from build123d import *

# Parameters (mm, degrees)
SKETCH1_W            = 70
SKETCH1_H            = 50
BOSS_EXTRUDE1_DEPTH  = 5
BOSS_EXTRUDE2_DEPTH  = 5
MIRROR2_COPY_1_DEPTH = 5


with BuildPart() as part:
    # Sketch1 → Boss-Extrude1 (new body)
    with BuildSketch(Plane.XY):
        Rectangle(SKETCH1_W, SKETCH1_H)
    extrude(amount=BOSS_EXTRUDE1_DEPTH)

    # Sketch2 → Boss-Extrude2 (add)
    with BuildSketch(Plane.ZY.offset(35)):
        Polygon((3.843440475, -25), (-7.895535709, -41.369324188), (-14.361094855, -42.788640383), (-29.004505052, -42.788640383), (-34.365162286, -38.4026481), (-35, -35), (-29.677149334, -39.79641498), (-19.61481892, -39.79641498), (-9.962095697, -37.111555615), (0, -24.21921522), align=None)
    boss_extrude2 = extrude(amount=-BOSS_EXTRUDE2_DEPTH)

    # Mirror1: Boss-Extrude2 across plane
    add(boss_extrude2.mirror(Plane.ZX))

    # Mirror2: Boss-Extrude2 across plane
    add(boss_extrude2.mirror(Plane(origin=(0, 0, 0), x_dir=(0, 0, 1), z_dir=(1, 0, 0))))

    # Mirror2 copy 1 sketch → Mirror2 copy 1 (add)
    with BuildSketch(Plane(origin=(35, 0, 0), x_dir=(0, 0, 1), z_dir=(1, 0, 0))):
        Polygon((3.843440475, -25), (-7.895535709, -41.369324188), (-14.361094855, -42.788640383), (-29.004505052, -42.788640383), (-34.365162286, -38.4026481), (-35, -35), (-29.677149334, -39.79641498), (-19.61481892, -39.79641498), (-9.962095697, -37.111555615), (0, -24.21921522), align=None)
    extrude(amount=-MIRROR2_COPY_1_DEPTH)


solid = part.part
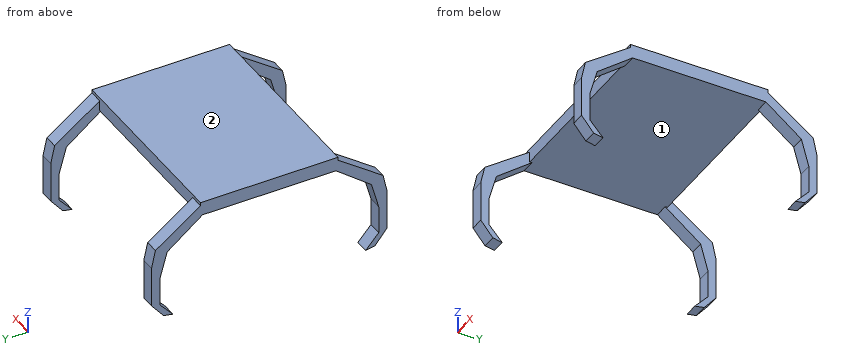
Model file for the job. Use its own axes, mm. Face numbers are marked on the shaded views. Coordinates: 2 decimals unless noted, no trailing zeros. Order: outer loops, then holes, each group sorted by start corner. A loop starts at its lowest first (then second) coordinate and runs counter-clockwise, first axis right, second up. Notation, with made-up numbers: M 2,-35 L 53,-35 A22 cw 53,-15 Z; hole C -23,-32 d5. An arc over 180 degrees is marked long. Return JSON: item names as keys, results as strings.
1. Flat gauge pins, fed straight in: pin 1 (1.5 mm diameter, centred on x = 5, z = 2, fed in from +Y); pin 2 (5.5 mm diameter, centred on x = 8.5, z = 3, fed in from -Y); pin 3 (8 mm diameter, centred on x = 15, y = -28.5, fed in from -Z). Where does each tip first touch, or does it go through?
Ans:
{"pin 1": "y = 25", "pin 2": "y = -25", "pin 3": "z = 0"}
2. Saw through at D-D (z = -9). Give the cut face in (x, y), and give its area (3 significant figures).
Ans:
{"outline": "M -35,-41.61 L -30,-41.61 L -30,-35.87 L -35,-35.87 Z; M -35,35.87 L -30,35.87 L -30,41.61 L -35,41.61 Z; M 30,-41.61 L 35,-41.61 L 35,-35.87 L 30,-35.87 Z; M 30,35.87 L 35,35.87 L 35,41.61 L 30,41.61 Z", "area": "115 mm^2"}
3. Drill centre lines: probe 1 along Z at (x, y) = (-32, 23); probe 2 along Y at (x, z) = (-28, 3); probe 3 along Y at (x, z) = (31, -3). Where is each one in solid material? Low to high.
Ans:
{"probe 1": "0 to 5", "probe 2": "-25 to 25", "probe 3": "-34.54 to -28.1, 28.1 to 34.54"}
4. Saw through at A-A (z = -27). Give the cut face in (x, y).
Ans:
{"outline": "M -35,-42.79 L -30,-42.79 L -30,-39.8 L -35,-39.8 Z; M -35,39.8 L -30,39.8 L -30,42.79 L -35,42.79 Z; M 30,-42.79 L 35,-42.79 L 35,-39.8 L 30,-39.8 Z; M 30,39.8 L 35,39.8 L 35,42.79 L 30,42.79 Z"}
5. Saw through at C-C (y = -3.5). Give the cut face in (x, z).
Ans:
{"outline": "M -35,0 L 35,0 L 35,5 L -35,5 Z"}
6. Pull direction Y, two halves, no side cores. Call the marked faces 1 and 2: +Y half, -Y half, draft (parallel to the pull), parting line (faces both ways), or undercut.
Ans:
{"face 1": "undercut", "face 2": "draft"}
7. Saw through at B-B (y = 33.5). Give the cut face in (x, z), and give its area (3 significant figures).
Ans:
{"outline": "M -35,-7.17 L -30,-7.17 L -30,-2.25 L -35,-2.25 Z; M 30,-7.17 L 35,-7.17 L 35,-2.25 L 30,-2.25 Z", "area": "49.2 mm^2"}
